from build123d import *

# Parameters (mm, degrees)
SKETCH1_W               = 125
SKETCH1_H               = 170
BOSS_EXTRUDE1_DEPTH     = 160
SKETCH2_R               = 3
CUT_EXTRUDE1_DEPTH      = 155
SKETCH2_3_R             = 3
CUT_EXTRUDE2_DEPTH      = 192.653985088
MIRROR2_COPY_1_SKETCH_R = 3
MIRROR2_COPY_1_DEPTH    = 155
MIRROR2_COPY_2_SKETCH_R = 3
MIRROR2_COPY_2_DEPTH    = 192.653985088


with BuildPart() as part:
    # Sketch1 → Boss-Extrude1 (new body)
    with BuildSketch(Plane.XY):
        Rectangle(SKETCH1_W, SKETCH1_H)
    extrude(amount=BOSS_EXTRUDE1_DEPTH)

    # Sketch2 → Cut-Extrude1 (cut)
    # profile 1 of 2: a face of its own
    with BuildSketch(Plane.XY.offset(160)):
        with BuildLine():
            Line((-50.5, 85), (-62.5, 85))
            Line((-62.5, 85), (-62.5, 73))
            Line((-62.5, 73), (-56.5, 73))
            ThreePointArc((-56.5, 73), (-52.257359313, 74.757359313), (-50.5, 79))
            Line((-50.5, 79), (-50.5, 85))
        make_face()
        with Locations((-56.5, 79)):
            Circle(SKETCH2_R, mode=Mode.SUBTRACT)
    # profile 2 of 2: a face of its own
    with BuildSketch(Plane.XY.offset(160)):
        with Locations((-56.5, 79)):
            Circle(SKETCH2_R)
    cut_extrude1 = extrude(amount=-CUT_EXTRUDE1_DEPTH, mode=Mode.SUBTRACT)

    # Sketch2<3> → Cut-Extrude2 (cut, through all)
    with BuildSketch(Plane.XY.offset(160)):
        with Locations((-56.5, 79)):
            Circle(SKETCH2_3_R)
    cut_extrude2 = extrude(amount=-CUT_EXTRUDE2_DEPTH, mode=Mode.SUBTRACT)

    # Mirror1: Cut-Extrude1, Cut-Extrude2 across plane
    add(cut_extrude1.mirror(Plane.ZX), mode=Mode.SUBTRACT)
    add(cut_extrude2.mirror(Plane.ZX), mode=Mode.SUBTRACT)

    # Mirror2: Cut-Extrude1, Cut-Extrude2 across plane
    add(cut_extrude1.mirror(Plane(origin=(0, 0, 0), x_dir=(0, 0, 1), z_dir=(1, 0, 0))), mode=Mode.SUBTRACT)
    add(cut_extrude2.mirror(Plane(origin=(0, 0, 0), x_dir=(0, 0, 1), z_dir=(1, 0, 0))), mode=Mode.SUBTRACT)

    # Mirror2 copy 1 sketch → Mirror2 copy 1 (cut)
    # profile 1 of 2: a face of its own
    with BuildSketch(Plane(origin=(0, 0, 160), x_dir=(-1, 0, 0), z_dir=(0, 0, 1))):
        with BuildLine():
            Line((-50.5, 85), (-62.5, 85))
            Line((-62.5, 85), (-62.5, 73))
            Line((-62.5, 73), (-56.5, 73))
            ThreePointArc((-56.5, 73), (-52.257359313, 74.757359313), (-50.5, 79))
            Line((-50.5, 79), (-50.5, 85))
        make_face()
        with Locations((-56.5, 79)):
            Circle(MIRROR2_COPY_1_SKETCH_R, mode=Mode.SUBTRACT)
    # profile 2 of 2: a face of its own
    with BuildSketch(Plane(origin=(0, 0, 160), x_dir=(-1, 0, 0), z_dir=(0, 0, 1))):
        with Locations((-56.5, 79)):
            Circle(MIRROR2_COPY_1_SKETCH_R)
    extrude(amount=-MIRROR2_COPY_1_DEPTH, mode=Mode.SUBTRACT)

    # Mirror2 copy 2 sketch → Mirror2 copy 2 (cut, through all)
    with BuildSketch(Plane(origin=(0, 0, 160), x_dir=(-1, 0, 0), z_dir=(0, 0, 1))):
        with Locations((-56.5, 79)):
            Circle(MIRROR2_COPY_2_SKETCH_R)
    extrude(amount=-MIRROR2_COPY_2_DEPTH, mode=Mode.SUBTRACT)


solid = part.part
The model under review builds one solid part; all positions refer to its coordinate system, in mm. A direction names the side the tool comes from. Coordinates: 2 decimals unless noted, no trailing zeros. Write each loop counter-clockwise with the first axis right and the second up, starting at its lowest first coordinate (ties: lowest second). Pieces come first, ordered by that corner, then holes. Notation, with made-up numbers: (52.5, 40.5) - (92.5, 40.5) arc R3 ccw to (92.5, 45.5) - close; hole circle Ø2 at (80, -19). An arc over 180 degrees is marked (long way). Answer as a JSON object with one key per item and string values. Group by question number.
1. To check wall thickness, follow probe 1 along Y at (x, z) = (56.5, 2.85); probe 2 along Z at (x, y) = (-56.5, -74.5); probe 3 along X at (y, z) = (73.5, 148). State the ranges of each line that lie inside material, in increasing order.
2. Mouldability with a two-part tool opening along Y and no side actions: class faces 6 (the face through (52.304, -74.711, 83.585)), 7 (the face through (-52.304, 74.711, 83.585)), 8 (the face through (58.9, -77.2, 2.5)) as pulls with the +Y half, pulls with the -Y half, needs draft (parallel to the pull), parting line crosses it, or undercut.
3. Clearance check with flat-ended pins moving along their axes: pin 1 Ø5.5 at (x, y) = (-56.5, -79) entering from +Z; pin 2 Ø3 at (x, z) = (58, 55) entering from -Y; pin 3 Ø3 at (y, z) = (-82, 111) entering from -X; pin 4 Ø6 at (x, y) = (54, -79.5) entering from +Z. State where each tip first meets the part, or that it passes through.
4. Add section A-A (z = 85). Give the boundary of the cut face in (x, y).
5. Machinability: for faces 1 (the face through (-62.5, -1, 79)), 2 (the face through (-58, 82, 5)), 3 (the face through (-52.304, -74.711, 83.585)), 4 (the face through (60, -73, 84)), 5 (the face through (50.5, 82, 84)), which of the approach directions +Z, -Z, +X, -X, +Y, -Y give a long, thin tool a straight path to every point of the face, cutting with its end or side? Answer none if there is none.
Findings:
{
 "1": {"probe 1": "-85 to -82, -76 to 76, 82 to 85", "probe 2": "0 to 5", "probe 3": "-54.1 to 54.1"},
 "2": {"face 6": "pulls with the -Y half", "face 7": "pulls with the +Y half", "face 8": "undercut"},
 "3": {"pin 1": "through", "pin 2": "y = -73", "pin 3": "x = -50.5", "pin 4": "z = 5"},
 "4": {"outline": "(-62.5, -73) - (-56.5, -73) arc R6 cw to (-50.5, -79) - (-50.5, -85) - (50.5, -85) - (50.5, -79) arc R6 cw to (56.5, -73) - (62.5, -73) - (62.5, 73) - (56.5, 73) arc R6 cw to (50.5, 79) - (50.5, 85) - (-50.5, 85) - (-50.5, 79) arc R6 cw to (-56.5, 73) - (-62.5, 73) - close"},
 "5": {"face 1": "+Z, -Z, -X, +Y, -Y", "face 2": "+Z, -X, +Y", "face 3": "+Z, -X, -Y", "face 4": "+Z, +X, -Y", "face 5": "+Z, +X, +Y"}
}
